Here's how the part is built. I have some questions about the finished solid (model axes, mm). Face numbers are marked on the shaded views. A direction names the side the tool comes from. Round coordinates to 2 decimals unless told otherwise and drop trailing zeros. Order: outer loops, then holes, each group sorted by start corner. A loop starts at its lowest first (then second) coordinate and runs counter-clockwise, first axis right, second up. Notation, with made-up numbers: (-4, 13.25) -> (14, 13.25) arc R21 ccw to (14, 27.25) -> close; hole circle Ø11 at (0.5, 57.25). An arc over 180 degrees is marked (long way). Use a Markdown table: item, result. Add a question column.
(1) Thinking about a two-plate mould opening in X: for the marked faces 3, 4 and 5, which applies, pulls with the +X half, pulls with the -X half, needs draft (parallel to the pull), parting line crosses it, or undercut?
(2) I want a section at C-C, the plane z = -5.5. Please give me the cut outline in (x, y), then the cut area to 3 significant figures.
(3) I want a section at A-A, the plane x = 0. Please give me the cut outline in (y, z).
(4) If I drill on probe 1 along X at (y, z) = (1.1, -5.5); probe 2 along X at (y, z) = (4.75, -2.25); probe 3 along Z at (x, y) = (2.5, 5.5), over which ranges is the centre line in solid material (lowest first)?
(5) I'm going to push flat-ended pins straight in: P1, Ø3.5, axis at x = -1.5, y = 6.5, coming from the -Z side; P2, Ø3.5, axis at x = 0, y = 5.5, coming from the +Z side; P3, Ø2, axis at x = -0.5, z = -6.5, coming from the +Y side. Where does each tip first touch, or does it pass through?
(6) I want a section at D-D, the plane y = 3.25. Please give me the cut outline in (x, z), then the cut area to 4 significant figures.
(7) I want a section at B-B, the plane y = 5.5. Please give me the cut outline in (x, z), then the cut area to 3 significant figures.
(8) On a 3-axis mill with a long thin cutter (end or side, diameter ignored), from which of +Z, -Z, +X, -X, +Y, -Y can I reach the whole of each face in a straight line? I mean the marked faces 1 and 2. Say none if no direction works.
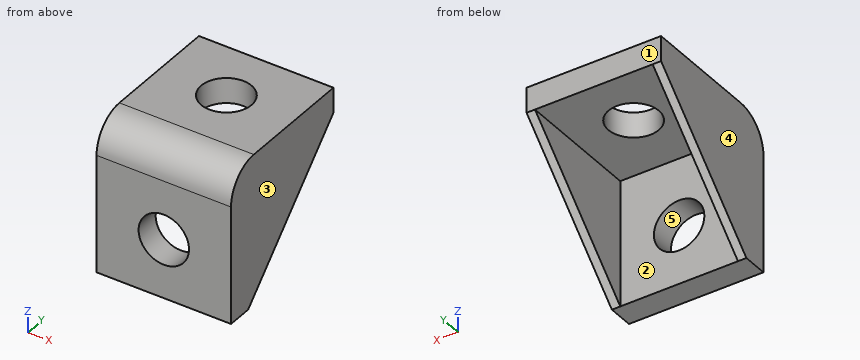
from build123d import *

# Parameters (mm, degrees)
BOSS_EXTRUDE1_DEPTH = 4
BOSS_EXTRUDE2_DEPTH = 0.5
SKETCH3_R           = 1.5
CUT_EXTRUDE1_DEPTH  = 14.341664064
SKETCH4_R           = 1.5
CUT_EXTRUDE2_DEPTH  = 14.341664064
FILLET1_R           = 2


with BuildPart() as part:
    # Sketch1 → Boss-Extrude1 (new, symmetric)
    with BuildSketch(Plane(origin=(0, 0, 0), x_dir=(0, 0, -1), z_dir=(1, 0, 0))):
        Polygon((0, 1.664846908), (0, 0), (1.75206606, 0), (9, 0), (9, 1.5), (1.5, 1.5), (1.5, 9), (0, 9), align=None)
    extrude(amount=BOSS_EXTRUDE1_DEPTH, both=True)

    # Sketch2 → Boss-Extrude2 (add)
    with BuildSketch(Plane(origin=(4, 0, 0), x_dir=(0, 0, -1), z_dir=(1, 0, 0))):
        Polygon((1.5, 9), (9, 1.5), (1.5, 1.5), align=None)
    boss_extrude2 = extrude(amount=-BOSS_EXTRUDE2_DEPTH)

    # Mirror1: Boss-Extrude2 across plane
    add(boss_extrude2.mirror(Plane(origin=(0, 0, 0), x_dir=(0, 0, 1), z_dir=(1, 0, 0))))

    # Sketch3 → Cut-Extrude1 (cut, through all)
    with BuildSketch(Plane.XY):
        with Locations((0, 5.5)):
            Circle(SKETCH3_R)
    extrude(amount=-CUT_EXTRUDE1_DEPTH, mode=Mode.SUBTRACT)

    # Sketch4 → Cut-Extrude2 (cut, through all)
    with BuildSketch(Plane.XZ):
        with Locations(Location((0, -5.5, 0), (0, 0, 270))):
            Circle(SKETCH4_R)
    extrude(amount=-CUT_EXTRUDE2_DEPTH, mode=Mode.SUBTRACT)

    # Fillet1
    fillet1_edges = [part.edges().sort_by_distance(p)[0] for p in [
        (0, 0, 0),
    ]]
    fillet(fillet1_edges, radius=FILLET1_R)


solid = part.part
Taken from the geometry:
| question | item | result |
|---|---|---|
| 1 | face 3 | pulls with the +X half |
| 1 | face 4 | pulls with the -X half |
| 1 | face 5 | undercut |
| 2 | outline | (-4, 0) -> (-1.5, 0) -> (-1.5, 1.5) -> (-3.5, 1.5) -> (-3.5, 5) -> (-4, 5) -> close; (1.5, 0) -> (4, 0) -> (4, 5) -> (3.5, 5) -> (3.5, 1.5) -> (1.5, 1.5) -> close |
| 2 | area | 11.0 mm2 |
| 3 | outline | (0, -9) -> (1.5, -9) -> (1.5, -7) -> (0, -7) -> close; (0, -4) -> (1.5, -4) -> (1.5, -1.5) -> (4, -1.5) -> (4, 0) -> (2, 0) arc R2 ccw to (0, -2) -> close; (7, -1.5) -> (9, -1.5) -> (9, 0) -> (7, 0) -> close |
| 4 | probe 1 | x = -4 to -1.5, 1.5 to 4 |
| 4 | probe 2 | x = -4 to -3.5, 3.5 to 4 |
| 4 | probe 3 | z = -1.5 to 0 |
| 5 | P1 | stops at z = -1.5 |
| 5 | P2 | stops at z = 0 |
| 5 | P3 | stops at y = 1.5 |
| 6 | outline | (-4, -7.25) -> (-3.5, -7.25) -> (-3.5, -1.5) -> (3.5, -1.5) -> (3.5, -7.25) -> (4, -7.25) -> (4, 0) -> (-4, 0) -> close |
| 6 | area | 17.75 mm2 |
| 7 | outline | (-4, -5) -> (-3.5, -5) -> (-3.5, -1.5) -> (-1.5, -1.5) -> (-1.5, 0) -> (-4, 0) -> close; (1.5, -1.5) -> (3.5, -1.5) -> (3.5, -5) -> (4, -5) -> (4, 0) -> (1.5, 0) -> close |
| 7 | area | 11.0 mm2 |
| 8 | face 1 | +Z, -Z, +X, -X, +Y |
| 8 | face 2 | -Z, +Y |
